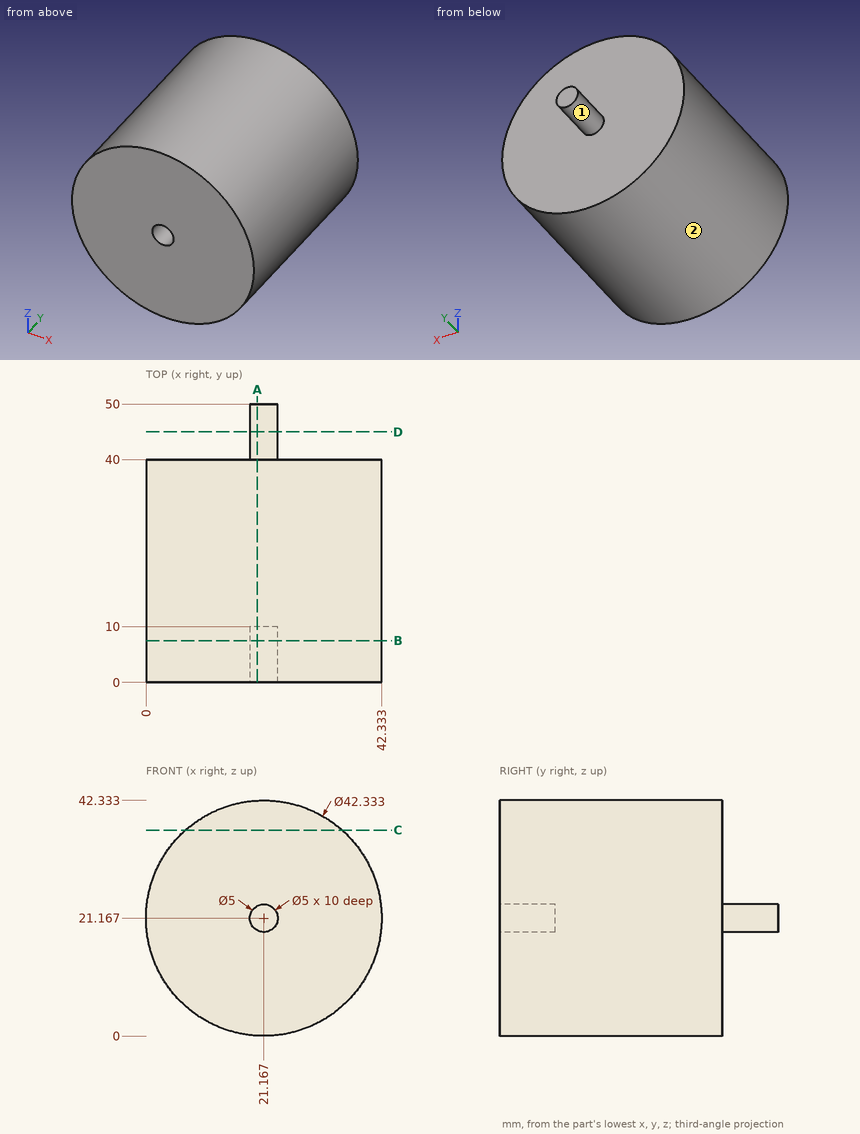
Geometry check sheet. Reference: drawing and pictorial views, mm from the part's lowest x, y, z. A direction names the side the tool comes from. Give positions to 0.01 mm unless a question says otherwise; leave off trailing zeros. Loops run counter-clockwise (first coordinate to the right, second up) from the corner with the lowest first, then second, coordinate; pieces in that order, holes last. Notation, with made-up numbers: M -40,-29 L -6,-29 A28 ccw -6,-8 Z; hole C 24.25,14.25 d5. An arc over 180 degrees is marked long. Use a Markdown table: item, result. Add a question column.
Q1. Sectioned sample at D-D, the plane y = 45. Record the cut outline in (x, z), then the cut area to 3 significant figures.
Q2. Go/stop test with flat-tipped pins: pin 1 (6 mm diameter, centred on x = 9.5, y = 8.5, fed in from -Z) (1 decimal); pin 2 (8 mm diameter, centred on y = 32, z = 18, fed in from -X); pin 3 (2 mm diameter, centred on x = 23.5, y = 45, fed in from +Z); pin 4 (2 mm diameter, centred on x = 6, y = 19, fed in from -Z). Record where each tip stops, or that it passes through.
Q3. Tool access check on the marked faces 1 and 2. Record the directions out of +Z, -Z, +X, -X, +Y, -Y that give a thin tool (end or side, any length) a straight path to the whole face; none if there is none.
Q4. Sectioned sample at A-A, the plane x = 20. Record the cut outline in (y, z) (1 decimal).
Q5. Scan lines: line 1 along Z through (x, y) = (21, 8); line 2 along Y through (x, z) = (24, 31.5); line 3 along Z through (x, y) = (20.5, 7). Record each from-to range of solid material in increasing order. Write a range as [from, to].
Q6. Sectioned sample at B-B, the plane y = 7.5. Record the cut outline in (x, z).
Q7. Sectioned sample at C-C, the plane z = 37. Record the cut outline in (x, y).
Verdict:
| question | item | result |
|---|---|---|
| 1 | outline | C 21.17,21.17 d5 |
| 1 | area | 19.6 mm^2 |
| 2 | pin 1 | z = 1.9 |
| 2 | pin 2 | x = 0 |
| 2 | pin 3 | z = 23.28 |
| 2 | pin 4 | z = 5.44 |
| 3 | face 1 | +Y |
| 3 | face 2 | +Y, -Y |
| 4 | outline | M 0,0 L 40,0 L 40,19 L 50,19 L 50,23.4 L 40,23.4 L 40,42.3 L 0,42.3 L 0,23.4 L 10,23.4 L 10,19 L 0,19 Z |
| 5 | line 1 | [0, 18.67], [23.66, 42.33] |
| 5 | line 2 | [0, 40] |
| 5 | line 3 | [0.01, 18.76], [23.58, 42.32] |
| 6 | outline | C 21.17,21.17 d42.33; hole C 21.17,21.17 d5 |
| 7 | outline | M 7.12,0 L 35.21,0 L 35.21,40 L 7.12,40 Z |
